CAD build for the part. Positions are in the model's coordinates, mm. Face numbers are marked on the shaded views. Round coordinates to 2 decimals unless told otherwise and drop trailing zeros. Order: outer loops, then holes, each group sorted by start corner. A loop starts at its lowest first (then second) coordinate and runs counter-clockwise, first axis right, second up. Notation, with made-up numbers: M 7.5,47 L 35.5,47 A14 cw 35.5,67 Z; hole C 53.25,-32.75 d10. An arc over 180 degrees is marked long. Answer as a JSON object with one key per item and string values. Group by question number.
```python
from build123d import *

# Parameters (mm, degrees)
SKETCH_W        = 150
SKETCH_H        = 150
PAD_DEPTH       = 4
POCKET_DEPTH    = 4.001
SKETCH002_R     = 1.9
SKETCH002_W     = 3.3
SKETCH002_H     = 64
SKETCH002_W_2   = 64
SKETCH002_H_2   = 3.3
POCKET001_DEPTH = 5
SKETCH003_R     = 2.95
POCKET002_DEPTH = 3
SKETCH004_W     = 10
SKETCH004_H     = 95
PAD001_DEPTH    = 11
POCKET003_DEPTH = 122.501
SKETCH006_R     = 3
POCKET004_DEPTH = 127.901


with BuildPart() as part:
    # Sketch → Pad (new body)
    with BuildSketch(Plane.XY):
        with Locations((75, 75)):
            Rectangle(SKETCH_W, SKETCH_H)
    extrude(amount=PAD_DEPTH)

    # Sketch001 (on Face6 of Pad) → Pocket (cut, through all)
    with BuildSketch(Plane.XY.offset(4)):
        Polygon((0, 110), (15, 110), (15, 135), (40, 135), (40, 150), (0, 150), align=None)
        Polygon((0, 40), (15, 40), (15, 15), (40, 15), (40, 0), (0, 0), align=None)
        Polygon((110, 150), (110, 135), (135, 135), (135, 110), (150, 110), (150, 150), align=None)
        Polygon((150, 40), (135, 40), (135, 15), (110, 15), (110, 0), (150, 0), align=None)
    extrude(amount=-POCKET_DEPTH, mode=Mode.SUBTRACT)

    # Sketch002 (on Face4 of Pocket) → Pocket001 (cut)
    with BuildSketch(Plane.XY.offset(4)):
        with Locations((18.9, 131.1)):
            Circle(SKETCH002_R)
        with Locations((131.1, 131.1)):
            Circle(SKETCH002_R)
        with Locations((131.1, 18.9)):
            Circle(SKETCH002_R)
        with Locations((18.9, 18.9)):
            Circle(SKETCH002_R)
        with Locations((4.65, 75)):
            Rectangle(SKETCH002_W, SKETCH002_H)
        with Locations((75, 145.35)):
            Rectangle(SKETCH002_W_2, SKETCH002_H_2)
        with Locations((145.35, 75)):
            Rectangle(SKETCH002_W, SKETCH002_H)
        with Locations((75, 4.65)):
            Rectangle(SKETCH002_W_2, SKETCH002_H_2)
    extrude(amount=-POCKET001_DEPTH, mode=Mode.SUBTRACT)

    # Sketch003 (on Face2 of Pocket001) → Pocket002 (cut)
    with BuildSketch(Plane(origin=(0, 0, 0), x_dir=(1, 0, 0), z_dir=(0, 0, -1))):
        with Locations((18.9, -131.1)):
            Circle(SKETCH003_R)
        with Locations((18.9, -18.9)):
            Circle(SKETCH003_R)
        with Locations((131.1, -18.9)):
            Circle(SKETCH003_R)
        with Locations((131.1, -131.1)):
            Circle(SKETCH003_R)
    extrude(amount=-POCKET002_DEPTH, mode=Mode.SUBTRACT)

    # Sketch004 (on Face4 of Pocket002) → Pad001 (join)
    with BuildSketch(Plane.XY.offset(4)):
        with Locations((27.1, 75)):
            Rectangle(SKETCH004_W, SKETCH004_H)
        with Locations((122.9, 75)):
            Rectangle(SKETCH004_W, SKETCH004_H)
    extrude(amount=PAD001_DEPTH)

    # Sketch005 (on Face52 of Pad001) → Pocket003 (cut, through all)
    with BuildSketch(Plane.XZ.offset(-27.5)):
        Polygon((24.96, 10), (32.1, 15), (32.1, 5), align=None)
        Polygon((117.9, 5), (125.04, 10), (117.9, 15), align=None)
    extrude(amount=-POCKET003_DEPTH, mode=Mode.SUBTRACT)

    # Sketch006 (on Face53 of Pocket003) → Pocket004 (cut, through all)
    with BuildSketch(Plane(origin=(22.1, 0, 0), x_dir=(0, -1, 0), z_dir=(-1, 0, 0))):
        with Locations((-42.7, 10)):
            Circle(SKETCH006_R)
    extrude(amount=-POCKET004_DEPTH, mode=Mode.SUBTRACT)


with BuildPart() as part_1:
    # Body placement: moved
    add(part.part.moved(Location((0, 0, -48))))


solid = part_1.part
```
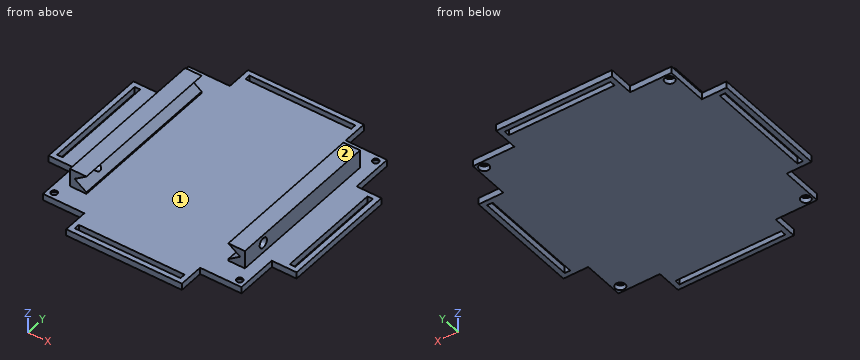
Item 1: Flat gauge pins, fed straight in: pin 1 Ø4.5 at (y, z) = (5.5, -47) entering from -X; pin 2 Ø3 at (x, y) = (20, 19) entering from -Z; pin 3 Ø1.2 at (x, z) = (126.5, -45.5) entering from -Y; pin 4 Ø1.2 at (x, z) = (59, -46) entering from -Y. Where does each tip first touch, or does it go through?
Item 2: Cut at C-C, the plane y = 131.1. Give the cut face in (x, z), and give its area (3 significant figures).
Item 3: Cut at A-A, the plane y = 98. Give the cut face in (x, z).
Item 4: Cut at B-B, the plane x = 51. Give the cut face in (y, z).
Item 5: Drill centre lines: line 1 (X direction, y = 93, z = -46.5); line 2 (X direction, y = 131.1, z = -44.25); line 3 (Y direction, x = 18.9, z = -45.9). Where is each one in solid material? Low to high. Write a range as [from, to].
Item 6: Two-plate mould, pull along X, no slides. Class the marked faces 1 and 2: +X half, -X half, draft (parallel to the pull), parting line (faces both ways), or undercut.
Response values:
{
 "1": {"pin 1": "x = 40", "pin 2": "z = -45", "pin 3": "y = 15", "pin 4": "y = 0"},
 "2": {"outline": "M 15,-48 L 15.95,-48 L 15.95,-45 L 17,-45 L 17,-44 L 15,-44 Z; M 20.8,-45 L 21.85,-45 L 21.85,-48 L 128.15,-48 L 128.15,-45 L 129.2,-45 L 129.2,-44 L 20.8,-44 Z; M 133,-45 L 134.05,-45 L 134.05,-48 L 135,-48 L 135,-44 L 133,-44 Z", "area": "437 mm^2"},
 "3": {"outline": "M 0,-48 L 3,-48 L 3,-44 L 0,-44 Z; M 6.3,-48 L 143.7,-48 L 143.7,-44 L 127.9,-44 L 127.9,-33 L 117.9,-33 L 125.04,-38 L 117.9,-43 L 117.9,-44 L 32.1,-44 L 32.1,-43 L 24.96,-38 L 32.1,-33 L 22.1,-33 L 22.1,-44 L 6.3,-44 Z; M 147,-48 L 150,-48 L 150,-44 L 147,-44 Z"},
 "4": {"outline": "M 0,-48 L 3,-48 L 3,-44 L 0,-44 Z; M 6.3,-48 L 143.7,-48 L 143.7,-44 L 6.3,-44 Z; M 147,-48 L 150,-48 L 150,-44 L 147,-44 Z"},
 "5": {"line 1": "[0, 3], [6.3, 143.7], [147, 150]", "line 2": "[15, 17], [20.8, 129.2], [133, 135]", "line 3": "[15, 15.95], [21.85, 128.15], [134.05, 135]"},
 "6": {"face 1": "undercut", "face 2": "draft"}
}
